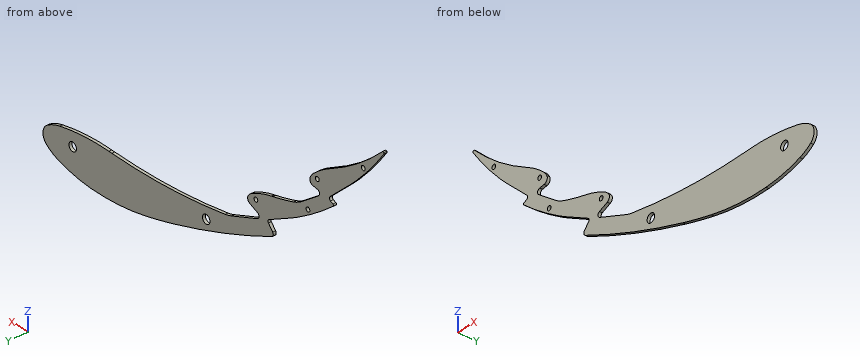
Autodesk Inventor part; units mm, degrees
ref_plane "YZ Plane" through (0, 0, 0) normal (1, 0, 0) x (0, 1, 0)
ref_plane "XZ Plane" through (0, 0, 0) normal (0, 1, 0) x (-1, 0, 0)
ref_plane "XY Plane" through (0, 0, 0) normal (0, 0, 1) x (1, 0, 0)
sketch "スケッチ1" plane through (0, 0, 0) normal (0, 1, 0) x (-1, 0, 0)
  arc A0 (352.9404, 45.4012) -> (350.2664, 52.9074) centre (351.268, 49.0348) ccw
  arc A1 (196.042, -12.8796) -> (352.9404, 45.4012) centre (-109.7603, 1050.7077) ccw
  arc A2 (150.312, -24.5744) -> (196.042, -12.8796) centre (-24.3171, 753.5344) ccw
  arc A3 (62.5903, -32.1265) -> (150.312, -24.5744) centre (78.6271, 294.8376) ccw
  arc A4 (7.8921, -21.3368) -> (62.5903, -32.1265) centre (71.9931, 159.5809) ccw
  arc A5 (-9.4003, -11.6891) -> (7.8921, -21.3368) centre (27.6212, 34.3463) ccw
  arc A6 (-8.119, 12.6128) -> (-9.4003, -11.6891) centre (0, 0) ccw
  arc A7 (11.7348, 20.8189) -> (-8.119, 12.6128) centre (24.3569, -37.8384) ccw
  arc A8 (90.7942, 27.108) -> (11.7348, 20.8189) centre (74.8452, -272.4677) ccw
  arc A9 (90.7942, 27.108) -> (95.7842, 26.8528) centre (154.5899, 1225.411) ccw
  arc A10 (95.7842, 26.8528) -> (350.2664, 52.9074) centre (137.4382, 875.8316) ccw
  arc A11 (451.6654, 129.0808) -> (449.8552, 131.7041) centre (450.6431, 130.3115) ccw
  arc A12 (397.0782, 90.3195) -> (451.6654, 129.0808) centre (168.8146, 469.5991) ccw
  arc A13 (380.6202, 81.0666) -> (397.0782, 90.3195) centre (232.593, 363.6259) ccw
  arc A14 (347.509, 69.0671) -> (380.6202, 81.0666) centre (319.8553, 197.0566) ccw
  arc A15 (325.2582, 67.5731) -> (347.509, 69.0671) centre (331.295, 144.1106) ccw
  arc A16 (317.5781, 69.5105) -> (325.2582, 67.5731) centre (327.1162, 91.13) ccw
  arc A17 (315.5573, 79.0327) -> (317.5781, 69.5105) centre (320, 75) ccw
  arc A18 (322.3786, 84.2587) -> (315.5573, 79.0327) centre (333.3281, 62.902) ccw
  arc A19 (352.2737, 94.8734) -> (322.3786, 84.2587) centre (377.1259, -22.5249) ccw
  arc A20 (352.2737, 94.8734) -> (354.2282, 95.2914) centre (252.865, 564.4668) ccw
  arc A21 (354.2282, 95.2914) -> (449.8552, 131.7041) centre (282.4293, 427.624) ccw
  arc A22 (533.1819, 231.3155) -> (533.0183, 233.3599) centre (531.8758, 232.2398) ccw
  arc A23 (490.4869, 179.7468) -> (533.1819, 231.3155) centre (171.8364, 487.0238) ccw
  arc A24 (476.9845, 166.5496) -> (490.4869, 179.7468) centre (260.8694, 401.1686) ccw
  arc A25 (448.1072, 146.3891) -> (476.9845, 166.5496) centre (388.2697, 262.8602) ccw
  arc A26 (427.0013, 139.1871) -> (448.1072, 146.3891) centre (413.023, 214.679) ccw
  arc A27 (419.0814, 139.0707) -> (427.0013, 139.1871) centre (422.699, 162.4222) ccw
  arc A28 (414.665, 147.7454) -> (419.0814, 139.0707) centre (420, 145) ccw
  arc A29 (419.9012, 154.5588) -> (414.665, 147.7454) centre (436.0051, 136.7638) ccw
  arc A30 (446.0304, 172.5493) -> (419.9012, 154.5588) centre (500.4207, 65.5835) ccw
  arc A31 (446.0304, 172.5493) -> (447.8101, 173.4589) centre (228.4693, 600.4128) ccw
  arc A32 (447.8101, 173.4589) -> (530.4702, 233.1021) centre (292.4437, 475.8846) ccw
  line L0 (530.4702, 233.1021) -> (525.5697, 238.1005)
  line L1 (525.5697, 238.1005) -> (526.9978, 239.5007)
  line L2 (526.9978, 239.5007) -> (533.0183, 233.3599)
  arc A33 (530.4702, 233.1021) -> (530.7544, 233.381) centre (292.4437, 475.8846) ccw
  arc A34 (533.0183, 233.3599) -> (530.7544, 233.381) centre (531.8758, 232.2398) ccw
  line L3 (317.5781, 69.5105) -> (338.9513, 60.0811)
  line L4 (338.9513, 60.0811) -> (283.0095, 38.3896)
  line L5 (380.6202, 81.0666) -> (345.1511, 62.485)
  line L6 (345.1511, 62.485) -> (354.3249, 51.6146)
  line L7 (419.0814, 139.0707) -> (435.7934, 136.4817)
  line L8 (435.7934, 136.4817) -> (395.4422, 106.9558)
  line L9 (476.9845, 166.5496) -> (443.1114, 135.348)
  line L10 (443.1114, 135.348) -> (451.2836, 131.7777)
  point P0 (0, 0)
  dimension "d2" = 45
  dimension "d3" = 45
  dimension "d4" = 60
  dimension "d5" = 50
extrude "押し出し1" add sketch "スケッチ1" along normal mid plane 4 contours A1 A2 A3 A4 A5 A6 A7 A8 A9 A10 A0 | A0 A10 L4 L3 A16 A15 A14 L5 L6 | A14 A15 A16 A17 A18 A19 A20 A21 A11 A12 A13 | A11 A21 L8 L7 A27 A26 A25 L9 L10 | A25 A26 A27 A28 A29 A30 A31 A32 A33 A34 A22 A23 A24
fillet "フィレット1" radius 4 2 edges at (-338.9513, 0, 60.0811) (-435.7934, 0, 136.4817)
fillet "フィレット1" radius 3 2 edges at (-443.1114, 0, 135.348) (-345.1511, 0, 62.485)
fillet "フィレット1" radius 50 2 edges at (-395.4422, 0, 106.9558) (-283.0095, 0, 38.3896)
sketch "スケッチ2" plane through (0, 2, 0) normal (0, 1, 0) x (1, 0, 0)
  circle A0 centre (-32.803, -5.2135) radius 6
  circle A1 centre (-247.4696, -17.1833) radius 6
  circle A2 centre (-327.3904, -78.8305) radius 3
  circle A3 centre (-411.0696, -106.0665) radius 3
  circle A4 centre (-426.1472, -150.6128) radius 3
  circle A5 centre (-499.9259, -198.5785) radius 3
  point P0 (0, 0)
extrude "押し出し2" cut sketch "スケッチ2" against normal through all
properties part number "bracket" material "木材 (オーク)"
Geometry: final body of the model. Coordinates: model frame, mm. Give positions to 0.01 mm unless a question says otherwise; leave off trailing zeros. Order: outer loops, then holes, each group sorted by start corner. A loop starts at its lowest first (then second) coordinate and runs counter-clockwise, first axis right, second up. Notation, with made-up numbers: (14, 49.25) -> (19, 49.25) arc R19 cw to (19, 59.25) -> close; hole circle Ø11 at (14.5, 83.5). An arc over 180 degrees is marked (long way). Put each result on its own line as item: value.
Q1. Section A-A, the plane y = 0. Count the separate pieces of the cut face and the enclosed holes in it, then the cut area to 3 significant figures.
Here are the results:
separate pieces: 1
enclosed holes: 6
area: 19,900 mm^2
Q2. Section C-C, the plane x = -458. Return loops of the section in (y, z), then the cut area to 3 significant figures.
Here are the results:
outline: (-2, 149.06) -> (2, 149.06) -> (2, 178.91) -> (-2, 178.91) -> close
area: 119 mm^2
Q3. Section B-B, the plane x = -57.5. Return loops of the section in (y, z), then the cut area to 3 significant figures.
Here are the results:
outline: (-2, -31.81) -> (2, -31.81) -> (2, 27.03) -> (-2, 27.03) -> close
area: 235 mm^2
Q4. Pin query (flat end, axial travel): pin 1 (7 mm diameter, centred on x = -327.39, z = 78.83, fed in from -Y); pin 2 (2 mm diameter, centred on x = -279, y = 0.5, fed in from +Z); pin 3 (2 mm diameter, centred on y = -0.5, z = 45, fed in from -X); pin 4 (2 mm diameter, centred on y = 0.5, z = 76.5, fed in from -X). Return the tip coordinate at first contact, or that it passes through.
Here are the results:
pin 1: stops at y = -2
pin 2: stops at z = 37.92
pin 3: stops at x = -353.87
pin 4: stops at x = -373.81
Q5. Material intervals for L1, parallel to X at y = 1.8, z = 77.5; L2, parallel to Z at x = -158, y = 1.5; L3, parallel to Z at x = -203.5, y = -0.55, sorted ascending.
Here are the results:
L1: x = -373.81 to -330.08, -324.7 to -314.55
L2: z = -22.81 to 26.08
L3: z = -10.71 to 28.4
